Input: dimensioned drawing with shaded views. Units: mm. Origin: part minimum x, y, z. A direction names the side the tool comes from. Round coordinates to 2 decimals unless told otherwise and drop trailing zeros. Write each loop counter-clockwise with the first axis right and the second up, starting at its lowest first coordinate (ties: lowest second). Pieces come first, ordered by that corner, then holes. Notation, with made-up numbers: M -1.5,28.5 L 34.5,28.5 A24 ccw 34.5,53.5 Z; hole C -0.5,88 d7. An arc over 180 degrees is marked long. Answer in a Markdown table with one row per item. Add a question column.
Item 1: Cut plane C-C on z = 14. Return loops of the section in (x, y).
Item 2: Mould query, pull axis X, two halves, no side actions, for the marked faces 1, 2 and 3. Classes: released by +X, released by -X, zero draft, split by the parting line, or undercut.
Item 3: Set-up query: the marked faces 4 and 5. Return all of +Z, -Z, +X, -X, +Y, -Y with unobstructed straight access to the full face (end or side cutting, diameter ignored); none if empty.
Item 4: Cut plane D-D on x = 54.5. Return loops of the section in (y, z).
Item 5: Cut plane A-A on x = 30. Return loops of the section in (y, z) (1 decimal).
Item 6: Material intervals for probe 1 along Z at (x, y) = (34, 47.5); probe 2 along Y at (x, z) = (30, 3.05) (1 decimal); probe 3 along Y at (x, z) = (28, 5.25), sorted ascending.
Item 7: Contact query for flat-ended pins moving along their axis: pin 1 (2.5 mm diameter, centred on x = 17.75, y = 8.78, fed in from +Z); pin 2 (1 mm diameter, centred on x = 8, z = 5, fed in from +Y); pin 3 (1.2 mm diameter, centred on x = 17.5, y = 50.5, fed in from -Z); pin 4 (6 mm diameter, centred on y = 9, z = 11.5, fed in from +X). Output: stop coordinate, or through.
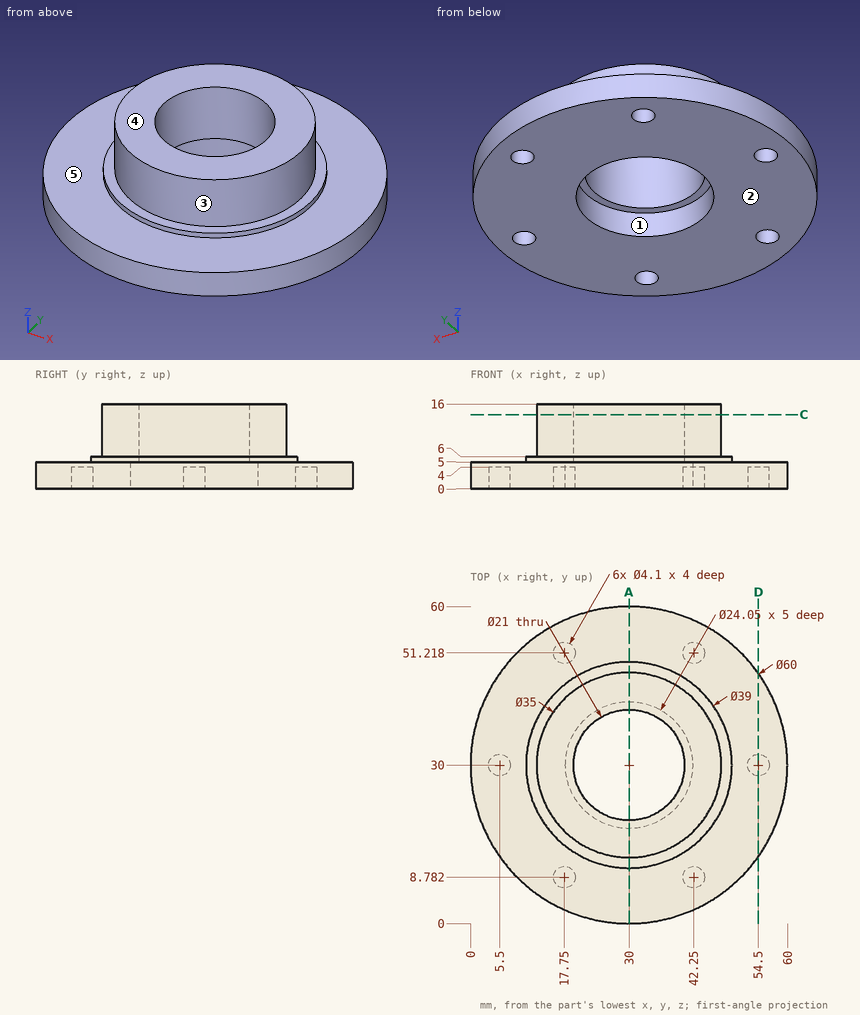
Results below:
| question | item | result |
|---|---|---|
| 1 | outline | C 30,30 d35; hole C 30,30 d21 |
| 2 | face 1 | undercut |
| 2 | face 2 | zero draft |
| 2 | face 3 | split by the parting line |
| 3 | face 4 | +Z, +X, -X, +Y, -Y |
| 3 | face 5 | +Z |
| 4 | outline | M 12.69,0 L 27.95,0 L 27.95,4 L 32.05,4 L 32.05,0 L 47.31,0 L 47.31,5 L 12.69,5 Z |
| 5 | outline | M 0,0 L 18,0 L 18,5 L 19.5,5 L 19.5,16 L 12.5,16 L 12.5,6 L 10.5,6 L 10.5,5 L 0,5 Z; M 40.5,5 L 42,5 L 42,0 L 60,0 L 60,5 L 49.5,5 L 49.5,6 L 47.5,6 L 47.5,16 L 40.5,16 Z |
| 6 | probe 1 | 0 to 6 |
| 6 | probe 2 | 0 to 18, 42 to 60 |
| 6 | probe 3 | 10.6 to 19.69, 40.31 to 49.4 |
| 7 | pin 1 | z = 5 |
| 7 | pin 2 | y = 50.92 |
| 7 | pin 3 | z = 4 |
| 7 | pin 4 | through |
